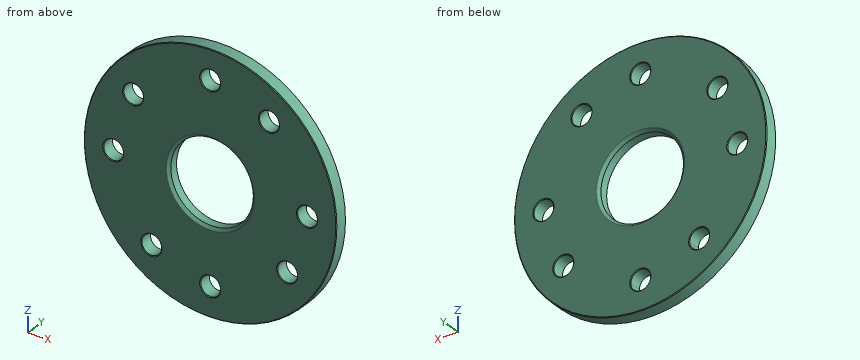
```python
from build123d import *

# Parameters (mm, degrees)
F0_R     = 92.5
F0_R_2   = 7.25
F0_R_3   = 30.25
F1_DEPTH = 10
F2_SIZE2 = 2
F2_SIZE  = 2
F3_SIZE2 = 2
F3_SIZE  = 2


# Not quite as in the source:
# - a fillet or chamfer that OpenCascade refuses, or shapes differently, is made with other operations: its cross-section is extruded or revolved along the edge and cut away or added


with BuildPart() as f1:
    # F0 (on Front) → F1 (new body)
    with BuildSketch(Plane.XZ):
        Circle(F0_R)
        with BuildLine():
            ThreePointArc((-35.8509998507, -56.4207746479), (-35.9472026921, -57.5979263852), (-36.2332581163, -58.7438380282))
            ThreePointArc((-36.2332581163, -58.7438380282), (-50.2547970094, -55.2436229106), (-35.8509998507, -56.4207746479))
        make_face(mode=Mode.SUBTRACT)
        with BuildLine():
            ThreePointArc((-6.8677417345, -68.6769366197), (1.1771517373, -63.8462028413), (7.25, -71))
            ThreePointArc((7.25, -71), (-1.1771517373, -78.1537971587), (-6.8677417345, -68.6769366197))
        make_face(mode=Mode.SUBTRACT)
        with Locations((56.4207746479, -43.1009998507)):
            Circle(F0_R_2, mode=Mode.SUBTRACT)
        with Locations((-71, 0)):
            Circle(F0_R_2, mode=Mode.SUBTRACT)
        with Locations((-56.4207746479, 43.1009998507)):
            Circle(F0_R_2, mode=Mode.SUBTRACT)
        Circle(F0_R_3, mode=Mode.SUBTRACT)
        with Locations((71, 0)):
            Circle(F0_R_2, mode=Mode.SUBTRACT)
        with Locations((43.1009998507, 56.4207746479)):
            Circle(F0_R_2, mode=Mode.SUBTRACT)
        with Locations((0, 71)):
            Circle(F0_R_2, mode=Mode.SUBTRACT)
    extrude(amount=-F1_DEPTH)

    # F2
    f2_edges = [f1.edges().sort_by_distance(p)[0] for p in [
        (-30.25, 0, 0),
    ]]
    chamfer(f2_edges, length=F2_SIZE, length2=F2_SIZE2)

    # F3
    f3_edges = [f1.edges().sort_by_distance(p)[0] for p in [
        (-30.25, 10, 0),
    ]]
    chamfer(f3_edges, length=F3_SIZE, length2=F3_SIZE2)

    # F4: chamfer of 0.5 on 10 edges, made by hand

    # F4_s1 → F4_t2 (revolve, cut)
    with BuildSketch(Plane.XY):
        Polygon((32.1035533906, 9.8535533906), (32.4571067812, 10), (32.25, 10), align=None)
    revolve(axis=Axis((0, 10, 0), (0, -1, 0)), mode=Mode.SUBTRACT)

    # F4_s3 → F4_t4 (revolve, cut)
    with BuildSketch(Plane.XY):
        Polygon((92, 10), (92.5, 9.5), (92.5, 10), align=None)
    revolve(axis=Axis((0, 10, 0), (0, -1, 0)), mode=Mode.SUBTRACT)

    # F4_s5 → F4_t6 (revolve, cut)
    with BuildSketch(Plane.XY.offset(-56.4207746479)):
        Polygon((-35.3509998507, 10), (-35.8509998507, 9.5), (-35.8509998507, 10), align=None)
    revolve(axis=Axis((-43.1009998507, 10, -56.4207746479), (0, 1, 0)), mode=Mode.SUBTRACT)

    # F4_s7 → F4_t8 (revolve, cut)
    with BuildSketch(Plane(origin=(-21.5504999254, 0, -63.7103873239), x_dir=(0, 1, 0), z_dir=(-0.3204225352, 0, -0.947274722))):
        Polygon((10, 15), (9.5, 15.5), (10, 15.5), align=None)
    revolve(axis=Axis((0, 10, -71), (0, 1, 0)), mode=Mode.SUBTRACT)

    # F4_s9 → F4_t10 (revolve, cut)
    with BuildSketch(Plane.XY.offset(-43.1009998507)):
        Polygon((64.1707746479, 10), (63.6707746479, 9.5), (63.6707746479, 10), align=None)
    revolve(axis=Axis((56.4207746479, 10, -43.1009998507), (0, -1, 0)), mode=Mode.SUBTRACT)

    # F4_s11 → F4_t12 (revolve, cut)
    with BuildSketch(Plane.XY):
        Polygon((-63.25, 10), (-63.75, 9.5), (-63.75, 10), align=None)
    revolve(axis=Axis((-71, 10, 0), (0, -1, 0)), mode=Mode.SUBTRACT)

    # F4_s13 → F4_t14 (revolve, cut)
    with BuildSketch(Plane.XY.offset(43.1009998507)):
        Polygon((-48.6707746479, 10), (-49.1707746479, 9.5), (-49.1707746479, 10), align=None)
    revolve(axis=Axis((-56.4207746479, 10, 43.1009998507), (0, -1, 0)), mode=Mode.SUBTRACT)

    # F4_s15 → F4_t16 (revolve, cut)
    with BuildSketch(Plane.XY):
        Polygon((78.75, 10), (78.25, 9.5), (78.25, 10), align=None)
    revolve(axis=Axis((71, 10, 0), (0, -1, 0)), mode=Mode.SUBTRACT)

    # F4_s17 → F4_t18 (revolve, cut)
    with BuildSketch(Plane.XY.offset(56.4207746479)):
        Polygon((50.8509998507, 10), (50.3509998507, 9.5), (50.3509998507, 10), align=None)
    revolve(axis=Axis((43.1009998507, 10, 56.4207746479), (0, -1, 0)), mode=Mode.SUBTRACT)

    # F4_s19 → F4_t20 (revolve, cut)
    with BuildSketch(Plane.XY.offset(71)):
        Polygon((7.75, 10), (7.25, 9.5), (7.25, 10), align=None)
    revolve(axis=Axis((0, 10, 71), (0, -1, 0)), mode=Mode.SUBTRACT)

    # F5: chamfer of 0.5 on 10 edges, made by hand

    # F5_s1 → F5_t2 (revolve, cut)
    with BuildSketch(Plane.XY):
        Polygon((32.1035533906, 0.1464466094), (32.4571067812, 0), (32.25, 0), align=None)
    revolve(axis=Axis((0, 0, 0), (0, -1, 0)), mode=Mode.SUBTRACT)

    # F5_s3 → F5_t4 (revolve, cut)
    with BuildSketch(Plane.XY):
        Polygon((92, 0), (92.5, 0.5), (92.5, 0), align=None)
    revolve(axis=Axis((0, 0, 0), (0, -1, 0)), mode=Mode.SUBTRACT)

    # F5_s5 → F5_t6 (revolve, cut)
    with BuildSketch(Plane.XY.offset(-56.4207746479)):
        Polygon((-35.3509998507, 0), (-35.8509998507, 0.5), (-35.8509998507, 0), align=None)
    revolve(axis=Axis((-43.1009998507, 0, -56.4207746479), (0, -1, 0)), mode=Mode.SUBTRACT)

    # F5_s7 → F5_t8 (revolve, cut)
    with BuildSketch(Plane(origin=(-21.5504999254, 0, -63.7103873239), x_dir=(0, 1, 0), z_dir=(0.3204225352, 0, 0.947274722))):
        Polygon((0, -15), (0.5, -15.5), (0, -15.5), align=None)
    revolve(axis=Axis((0, 0, -71), (0, -1, 0)), mode=Mode.SUBTRACT)

    # F5_s9 → F5_t10 (revolve, cut)
    with BuildSketch(Plane.XY.offset(-43.1009998507)):
        Polygon((64.1707746479, 0), (63.6707746479, 0.5), (63.6707746479, 0), align=None)
    revolve(axis=Axis((56.4207746479, 0, -43.1009998507), (0, -1, 0)), mode=Mode.SUBTRACT)

    # F5_s11 → F5_t12 (revolve, cut)
    with BuildSketch(Plane.XY):
        Polygon((-63.25, 0), (-63.75, 0.5), (-63.75, 0), align=None)
    revolve(axis=Axis((-71, 0, 0), (0, -1, 0)), mode=Mode.SUBTRACT)

    # F5_s13 → F5_t14 (revolve, cut)
    with BuildSketch(Plane.XY.offset(43.1009998507)):
        Polygon((-48.6707746479, 0), (-49.1707746479, 0.5), (-49.1707746479, 0), align=None)
    revolve(axis=Axis((-56.4207746479, 0, 43.1009998507), (0, -1, 0)), mode=Mode.SUBTRACT)

    # F5_s15 → F5_t16 (revolve, cut)
    with BuildSketch(Plane.XY):
        Polygon((78.75, 0), (78.25, 0.5), (78.25, 0), align=None)
    revolve(axis=Axis((71, 0, 0), (0, -1, 0)), mode=Mode.SUBTRACT)

    # F5_s17 → F5_t18 (revolve, cut)
    with BuildSketch(Plane.XY.offset(56.4207746479)):
        Polygon((50.8509998507, 0), (50.3509998507, 0.5), (50.3509998507, 0), align=None)
    revolve(axis=Axis((43.1009998507, 0, 56.4207746479), (0, -1, 0)), mode=Mode.SUBTRACT)

    # F5_s19 → F5_t20 (revolve, cut)
    with BuildSketch(Plane.XY.offset(71)):
        Polygon((7.75, 0), (7.25, 0.5), (7.25, 0), align=None)
    revolve(axis=Axis((0, 0, 71), (0, -1, 0)), mode=Mode.SUBTRACT)


solid = f1.part
```
Check sheet for the modelled part. Datum: model origin and axes. Units: mm. Coordinates: 2 decimals unless noted, no trailing zeros. Write each question's results on one line, items separated by ' | '. Start each with the question number.
1) Depth check by flat-ended pin: pin 1 (11.5 mm diameter, centred on x = -56.42, z = 43.1, fed in from +Y); pin 2 (1.5 mm diameter, centred on y = 8.5, z = 33.5, fed in from +X); pin 3 (2 mm diameter, centred on y = 8, z = 58, fed in from +X); pin 4 (3 mm diameter, centred on y = 7.5, z = -8.5, fed in from -X). Enter the tip coordinate at first touch or a pass-through.
2) Material ranges on line 1 along Z through (x, y) = (49, 3.75); line 2 along Z through (x, y) = (-71, 5); line 3 along X through (y, z) = (2.75, 13), recorded low to high.
3) Section check A-A (y = 4.75). Count the separate pieces of the cut face and the enclosed holes in it, and give its area (3 significant figures).
Checked values:
1) pin 1: through | pin 2: x = 86.51 | pin 3: x = 72.85 | pin 4: x = -92.23
2) line 1: -78.46 to 52.21, 60.64 to 78.46 | line 2: -59.29 to -7.25, 7.25 to 59.29 | line 3: -91.58 to -27.31, 27.31 to 91.58
3) separate pieces: 1 | enclosed holes: 9 | area: 22,700 mm²
